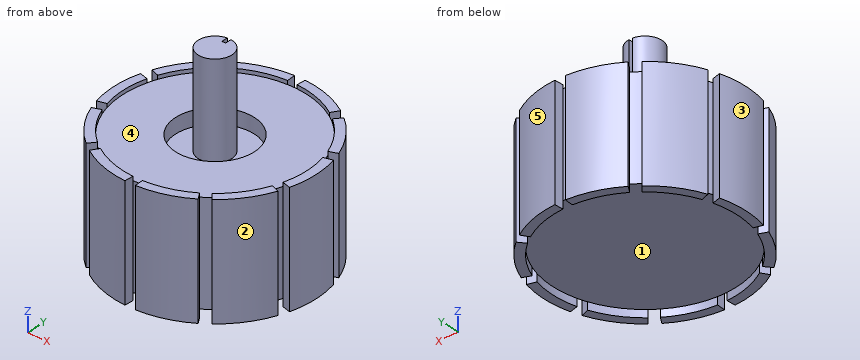
```python
from build123d import *

# Parameters (mm, degrees)
SKETCH1_R           = 24.5
BOSS_EXTRUDE1_DEPTH = 30
SKETCH2_R           = 10.491597787
CUT_EXTRUDE1_DEPTH  = 5
BOSS_EXTRUDE3_DEPTH = 30
SKETCH6_R           = 24.5
CUT_EXTRUDE2_DEPTH  = 2
SKETCH7_R           = 24.5
CUT_EXTRUDE4_DEPTH  = 1
SKETCH4_R           = 4.5
BOSS_EXTRUDE4_DEPTH = 25
CUT_EXTRUDE5_DEPTH  = 14


with BuildPart() as part:
    # Sketch1 → Boss-Extrude1 (new body)
    with BuildSketch(Plane.XY):
        Circle(SKETCH1_R)
    extrude(amount=BOSS_EXTRUDE1_DEPTH)

    # Sketch2 → Cut-Extrude1 (cut)
    with BuildSketch(Plane.XY.offset(30)):
        Circle(SKETCH2_R)
    extrude(amount=-CUT_EXTRUDE1_DEPTH, mode=Mode.SUBTRACT)

    # Sketch5 → Boss-Extrude3 (add)
    with BuildSketch(Plane(origin=(0, 0, 0), x_dir=(-1, 0, 0), z_dir=(0, 0, -1))):
        with BuildLine():
            ThreePointArc((-1.28221594, -24.466424387), (-7.570916362, -23.300884649), (-13.343668945, -20.54742074))
            Line((-13.343668945, -20.54742074), (-14.650803863, -22.560229302))
            ThreePointArc((-14.650803863, -22.560229302), (-8.312557149, -25.583420288), (-1.407820766, -26.863135347))
            Line((-1.407820766, -26.863135347), (-1.28221594, -24.466424387))
        make_face()
        with BuildLine():
            ThreePointArc((13.343668945, -20.54742074), (7.570916362, -23.300884649), (1.28221594, -24.466424387))
            Line((1.28221594, -24.466424387), (1.407820766, -26.863135347))
            ThreePointArc((1.407820766, -26.863135347), (8.312557149, -25.583420288), (14.650803863, -22.560229302))
            Line((14.650803863, -22.560229302), (13.343668945, -20.54742074))
        make_face()
        with BuildLine():
            ThreePointArc((22.872725828, -8.780000752), (19.820916362, -14.400738681), (15.418337917, -19.040085501))
            Line((15.418337917, -19.040085501), (16.928705712, -20.905236734))
            ThreePointArc((16.928705712, -20.905236734), (21.762557149, -15.811423287), (25.113319378, -9.640082458))
            Line((25.113319378, -9.640082458), (22.872725828, -8.780000752))
        make_face()
        with BuildLine():
            Line((25.983400462, 6.962248231), (23.665178859, 6.341081103))
            ThreePointArc((23.665178859, 6.341081103), (24.290398124, 3.19789915), (24.5, 0))
            ThreePointArc((24.5, 0), (24.290398124, -3.19789915), (23.665178859, -6.341081103))
            Line((23.665178859, -6.341081103), (25.983400462, -6.962248231))
            ThreePointArc((25.983400462, -6.962248231), (26.9, 0), (25.983400462, 6.962248231))
        make_face()
        with BuildLine():
            Line((16.928705712, 20.905236734), (15.418337917, 19.040085501))
            ThreePointArc((15.418337917, 19.040085501), (19.820916362, 14.400738681), (22.872725828, 8.780000752))
            Line((22.872725828, 8.780000752), (25.113319378, 9.640082458))
            ThreePointArc((25.113319378, 9.640082458), (21.762557149, 15.811423287), (16.928705712, 20.905236734))
        make_face()
        with BuildLine():
            Line((1.407820766, 26.863135347), (1.28221594, 24.466424387))
            ThreePointArc((1.28221594, 24.466424387), (7.570916362, 23.300884649), (13.343668945, 20.54742074))
            Line((13.343668945, 20.54742074), (14.650803863, 22.560229302))
            ThreePointArc((14.650803863, 22.560229302), (8.312557149, 25.583420288), (1.407820766, 26.863135347))
        make_face()
        with BuildLine():
            Line((-14.650803863, 22.560229302), (-13.343668945, 20.54742074))
            ThreePointArc((-13.343668945, 20.54742074), (-7.570916362, 23.300884649), (-1.28221594, 24.466424387))
            Line((-1.28221594, 24.466424387), (-1.407820766, 26.863135347))
            ThreePointArc((-1.407820766, 26.863135347), (-8.312557149, 25.583420288), (-14.650803863, 22.560229302))
        make_face()
        with BuildLine():
            Line((-25.113319378, 9.640082458), (-22.872725828, 8.780000752))
            ThreePointArc((-22.872725828, 8.780000752), (-19.820916362, 14.400738681), (-15.418337917, 19.040085501))
            Line((-15.418337917, 19.040085501), (-16.928705712, 20.905236734))
            ThreePointArc((-16.928705712, 20.905236734), (-21.762557149, 15.811423287), (-25.113319378, 9.640082458))
        make_face()
        with BuildLine():
            ThreePointArc((-23.665178859, -6.341081103), (-24.5, 0), (-23.665178859, 6.341081103))
            Line((-23.665178859, 6.341081103), (-25.983400462, 6.962248231))
            ThreePointArc((-25.983400462, 6.962248231), (-26.9, 0), (-25.983400462, -6.962248231))
            Line((-25.983400462, -6.962248231), (-23.665178859, -6.341081103))
        make_face()
        with BuildLine():
            ThreePointArc((-15.418337917, -19.040085501), (-19.820916362, -14.400738681), (-22.872725828, -8.780000752))
            Line((-22.872725828, -8.780000752), (-25.113319378, -9.640082458))
            ThreePointArc((-25.113319378, -9.640082458), (-21.762557149, -15.811423287), (-16.928705712, -20.905236734))
            Line((-16.928705712, -20.905236734), (-15.418337917, -19.040085501))
        make_face()
    extrude(amount=-BOSS_EXTRUDE3_DEPTH)

    # Sketch6 → Cut-Extrude2 (cut)
    with BuildSketch(Plane(origin=(0, 0, 0), x_dir=(-1, 0, 0), z_dir=(0, 0, -1))):
        Circle(SKETCH6_R)
    extrude(amount=-CUT_EXTRUDE2_DEPTH, mode=Mode.SUBTRACT)

    # Sketch7 → Cut-Extrude4 (cut)
    with BuildSketch(Plane.XY.offset(30)):
        Circle(SKETCH7_R)
    extrude(amount=-CUT_EXTRUDE4_DEPTH, mode=Mode.SUBTRACT)

    # Sketch4 → Boss-Extrude4 (add)
    with BuildSketch(Plane.XY.offset(25)):
        Circle(SKETCH4_R)
    extrude(amount=BOSS_EXTRUDE4_DEPTH)

    # Sketch8 → Cut-Extrude5 (cut)
    with BuildSketch(Plane.XY.offset(50)):
        with BuildLine():
            Line((-0.5, 2.742191979), (0.5, 2.742191979))
            Line((0.5, 2.742191979), (0.5, 4.472135955))
            ThreePointArc((0.5, 4.472135955), (0, 4.5), (-0.5, 4.472135955))
            Line((-0.5, 4.472135955), (-0.5, 2.742191979))
        make_face()
    extrude(amount=-CUT_EXTRUDE5_DEPTH, mode=Mode.SUBTRACT)


solid = part.part
```
Design review of the part built by this model. Coordinates are the model's own, in mm. Face numbers are marked on the shaded views. A direction names the side the tool comes from. Coordinates: 2 decimals unless noted, no trailing zeros. Loops run counter-clockwise (first coordinate to the right, second up) from the corner with the lowest first, then second, coordinate; pieces in that order, holes last. Notation, with made-up numbers: (50, -33) - (98, -33) arc R24 ccw to (98, 2) - close; hole circle Ø10 at (16.25, -2.5). An arc over 180 degrees is marked (long way). Use CSV: the item, a comma, the result in double quotes. Start each with the question number.
1) For pin 1 Ø1.6 at (x, y) = (25.5, -2.5) entering from +Z; pin 2 Ø10 at (x, z) = (11.5, 22.5) entering from -Y; pin 3 Ø12 at (x, z) = (19, 13.5) entering from -Y; pin 4 Ø8 at (y, z) = (12, 39.5) entering from +X, all flat-tipped, find the tip position at first contact; note any pin that passes through.
2) Wall thickness on L1, parallel to Y at x = 0, z = 28; L2, parallel to Y at x = 19, z = 20.5; L3, parallel to Z at x = -1, y = -19: over which ranges is each line inside the solid? List them lowest first. Write a range as from..to.
3) Consider section A-A on y = 0. Write out the cut boundary in (x, z), then the cut area to 3 significant figures.
4) Consider section C-C on y = -14. Write out the cut boundary in (x, z).
5) The part is to be moulded in two halves that separate along Y. For the marked faces 1, 2 and 3, say which applies: +Y half, -Y half, draft (parallel to the pull), parting line (faces both ways), or undercut.
6) Consider section B-B on x = -19. Write out the cut boundary in (y, z), then the cut area to 3 significant figures.
7) Tool access review of the marked faces 4 and 5: name each direction out of +Z, -Z, +X, -X, +Y, -Y from which nothing blocks a thin tool from reaching the whole face with its end or side.
Geometry says:
1,pin 1,"z = 30"
1,pin 2,"y = -26.1"
1,pin 3,"y = -23.55"
1,pin 4,"through"
2,L1,"-24.5..-10.49, -4.5..4.5, 10.49..24.5"
2,L2,"-19.04..19.04"
2,L3,"2..29"
3,outline,"(-26.9, 0) - (-24.5, 0) - (-24.5, 2) - (24.5, 2) - (24.5, 0) - (26.9, 0) - (26.9, 30) - (24.5, 30) - (24.5, 29) - (10.49, 29) - (10.49, 25) - (4.5, 25) - (4.5, 50) - (-4.5, 50) - (-4.5, 25) - (-10.49, 25) - (-10.49, 29) - (-24.5, 29) - (-24.5, 30) - (-26.9, 30) - close"
3,area,"1,610 mm^2"
4,outline,"(-22.97, 0) - (-20.11, 0) - (-20.11, 2) - (20.11, 2) - (20.11, 0) - (22.97, 0) - (22.97, 30) - (20.11, 30) - (20.11, 29) - (-20.11, 29) - (-20.11, 30) - (-22.97, 30) - close"
5,face 1,"undercut"
5,face 2,"-Y half"
5,face 3,"parting line"
6,outline,"(-19.04, 0) - (-15.47, 0) - (-15.47, 2) - (15.47, 2) - (15.47, 0) - (19.04, 0) - (19.04, 30) - (15.47, 30) - (15.47, 29) - (-15.47, 29) - (-15.47, 30) - (-19.04, 30) - close"
6,area,"1,050 mm^2"
7,face 4,"+Z"
7,face 5,"+Z, -Z, +X, +Y"
